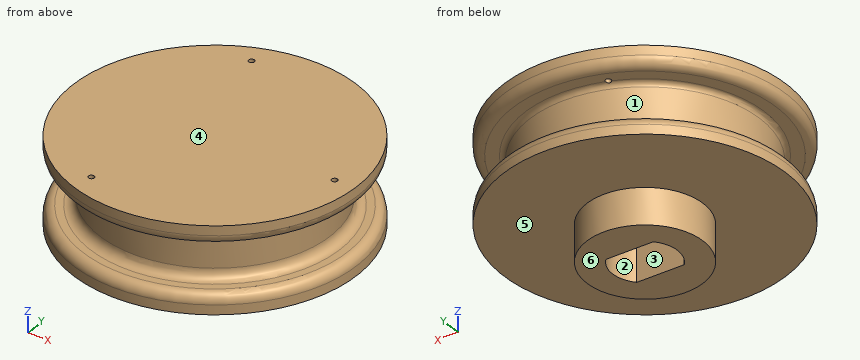
from build123d import *

# Parameters (mm, degrees)
SKETCH1_R           = 14.799242092
BOSS_EXTRUDE1_DEPTH = 2
SKETCH2_R           = 12.023378779
BOSS_EXTRUDE2_DEPTH = 5
SKETCH3_R           = 14.798614579
BOSS_EXTRUDE3_DEPTH = 2
SKETCH4_R           = 6.085537025
BOSS_EXTRUDE5_DEPTH = 3.8
FILLET5_R           = 1
FILLET6_R           = 0.5
CUT_EXTRUDE1_DEPTH  = 8.3
SKETCH8_R           = 0.302475122
SKETCH8_R_2         = 0.3
CUT_EXTRUDE3_DEPTH  = 2.3
FILLET7_R           = 1
FILLET8_R           = 1


with BuildPart() as part:
    # Sketch1 → Boss-Extrude1 (new body)
    with BuildSketch(Plane.XY):
        Circle(SKETCH1_R)
    extrude(amount=BOSS_EXTRUDE1_DEPTH)

    # Sketch2 → Boss-Extrude2 (add)
    with BuildSketch(Plane(origin=(0, 0, 0), x_dir=(-1, 0, 0), z_dir=(0, 0, -1))):
        Circle(SKETCH2_R)
    extrude(amount=BOSS_EXTRUDE2_DEPTH)

    # Sketch3 → Boss-Extrude3 (add)
    with BuildSketch(Plane(origin=(0, 0, -5), x_dir=(-1, 0, 0), z_dir=(0, 0, -1))):
        Circle(SKETCH3_R)
    extrude(amount=BOSS_EXTRUDE3_DEPTH)

    # Sketch4 → Boss-Extrude5 (add)
    with BuildSketch(Plane(origin=(0, 0, -7), x_dir=(-1, 0, 0), z_dir=(0, 0, -1))):
        with Locations(Location((0, 0, 0), (0, 0, 180))):
            Circle(SKETCH4_R)
    extrude(amount=BOSS_EXTRUDE5_DEPTH)

    # Fillet5
    fillet5_edges = [part.edges().sort_by_distance(p)[0] for p in [
        (-14.799242092, 0, 0),
    ]]
    fillet(fillet5_edges, radius=FILLET5_R)

    # Fillet6
    fillet6_edges = [part.edges().sort_by_distance(p)[0] for p in [
        (12.023378779, 0, 0),
    ]]
    fillet(fillet6_edges, radius=FILLET6_R)

    # Sketch7 → Cut-Extrude1 (cut)
    with BuildSketch(Plane(origin=(0, 0, -10.8), x_dir=(-1, 0, 0), z_dir=(0, 0, -1))):
        with BuildLine():
            Line((0, -2.3), (-2.503996805, -2.3))
            ThreePointArc((-2.503996805, -2.3), (-3.4, 0), (-2.503996805, 2.3))
            Line((-2.503996805, 2.3), (0, 2.3))
            Line((0, 2.3), (2.503996805, 2.3))
            ThreePointArc((2.503996805, 2.3), (3.4, 0), (2.503996805, -2.3))
            Line((2.503996805, -2.3), (0, -2.3))
        make_face()
    extrude(amount=-CUT_EXTRUDE1_DEPTH, mode=Mode.SUBTRACT)

    # Sketch8 → Cut-Extrude3 (cut)
    with BuildSketch(Plane.XY.offset(2)):
        with Locations((12.610771715, 0)):
            Circle(SKETCH8_R)
        with Locations((-4.484302396, 11.786542974)):
            Circle(SKETCH8_R_2)
        with Locations((-4.755704429, -11.679676307)):
            Circle(SKETCH8_R_2)
    extrude(amount=-CUT_EXTRUDE3_DEPTH, mode=Mode.SUBTRACT)

    # Fillet7
    fillet7_edges = [part.edges().sort_by_distance(p)[0] for p in [
        (12.023378779, 0, -5),
    ]]
    fillet(fillet7_edges, radius=FILLET7_R)

    # Fillet8
    fillet8_edges = [part.edges().sort_by_distance(p)[0] for p in [
        (14.798614579, 0, -5),
    ]]
    fillet(fillet8_edges, radius=FILLET8_R)


solid = part.part
Build history of the part. All positions in model axes, mm. Face numbers are marked on the shaded views. A direction names the side the tool comes from. Give positions to 0.01 mm unless a question says otherwise; leave off trailing zeros. Loops run counter-clockwise (first coordinate to the right, second up) from the corner with the lowest first, then second, coordinate; pieces in that order, holes last. Notation, with made-up numbers: (-5.5, 66.25) - (48.5, 66.25) arc R35 ccw to (48.5, 98.25) - close; hole circle Ø6 at (1.25, 42.5). An arc over 180 degrees is marked (long way). Write item = value, one per line. Start each with the question number.
1) Drop flat-ended pins along their axis: pin 1 Ø6 at (x, z) = (11, 0.5) entering from -Y; pin 2 Ø2.5 at (x, z) = (-0.5, -8.5) entering from +Y; pin 3 Ø2 at (x, y) = (-11.5, 2) entering from -Z. Give the stop position or say it passes through.
2) Tool access for the marked faces 5 and 6: list every direction of +Z, -Z, +X, -X, +Y, -Y with a clear straight run to the whole face (end or side of a thin tool).
3) Band-saw the part on C-C on z = -1. Give the cut face in (x, y), plus the area to 3 significant figures.
4) Pull direction X, two halves, no side cores. Call the marked faces 1, 2, 3 and 4: +X half, -X half, draft (parallel to the pull), parting line (faces both ways), or undercut.
5) Band-saw the part on B-B on x = 0. Give the cut face in (y, z), plus the area to 3 significant figures.
6) Probe probe 1 along Y at (x, z) = (-0.25, -10); probe 2 along Z at (x, y) = (4.25, 8.25); probe 3 along Z at (x, y) = (7.5, -11). List the from-to ranges inside material, lowest first. Write a range as from..to.
7) Band-saw the part on A-A on z = -9.5. Give the cut face in (x, y), plus the area to 3 significant figures.
Final values:
q1.pin_1 = -12.43
q1.pin_2 = 6.09
q1.pin_3 = -7
q2.face_5 = -Z
q2.face_6 = -Z, +X, -X, +Y, -Y
q3.outline = circle Ø24.05 at (0, 0)
q3.area = 454 mm²
q4.face_1 = parting line
q4.face_2 = undercut
q4.face_3 = undercut
q4.face_4 = draft
q5.outline = (-14.8, -7) - (-6.09, -7) - (-6.09, -10.8) - (-2.3, -10.8) - (-2.3, -2.5) - (2.3, -2.5) - (2.3, -10.8) - (6.09, -10.8) - (6.09, -7) - (14.8, -7) - (14.8, -6) arc R1 ccw to (13.8, -5) - (13.02, -5) arc R1 cw to (12.02, -4) - (12.02, -0.5) arc R0.5 cw to (12.52, 0) - (13.8, 0) arc R1 ccw to (14.8, 1) - (14.8, 2) - (-14.8, 2) - (-14.8, 1) arc R1 ccw to (-13.8, 0) - (-12.52, 0) arc R0.5 cw to (-12.02, -0.5) - (-12.02, -4) arc R1 cw to (-13.02, -5) - (-13.8, -5) arc R1 ccw to (-14.8, -6) - close
q5.area = 246 mm²
q6.probe_1 = -6.08..-2.3, 2.3..6.08
q6.probe_2 = -7..2
q6.probe_3 = -7..-5, 0..2
q7.outline = circle Ø12.17 at (0, 0); hole (-2.5, -2.3) - (2.5, -2.3) arc R3.4 ccw to (2.5, 2.3) - (-2.5, 2.3) arc R3.4 ccw to start
q7.area = 87.6 mm²
